Here's how the part is built. I have some questions about the finished solid (model axes, mm). Round coordinates to 2 decimals unless told otherwise and drop trailing zeros. Write each loop counter-clockwise with the first axis right and the second up, starting at its lowest first coordinate (ties: lowest second). Pieces come first, ordered by that corner, then holes. Notation, with made-up numbers: (46.25, -12) -> (92.25, -12) arc R19 cw to (92.25, 3) -> close; hole circle Ø5 at (60, 67.5). An arc over 180 degrees is marked (long way). Answer in a Markdown table with one row per item.
Autodesk Inventor part; units mm, degrees
ref_plane "YZ Plane" through (0, 0, 0) normal (1, 0, 0) x (0, 1, 0)
ref_plane "XZ Plane" through (0, 0, 0) normal (0, 1, 0) x (-1, 0, 0)
ref_plane "XY Plane" through (0, 0, 0) normal (0, 0, 1) x (1, 0, 0)
sketch "Sketch1" plane through (0, 0, 0) normal (0, 0, 1) x (1, 0, 0)
  line L0 (0, 0) -> (425, 0)
  line L1 (425, 0) -> (425, 300)
  line L2 (425, 300) -> (0, 300)
  line L3 (0, 300) -> (0, 0)
  line L4 (12.5, 287.5) -> (12.5, 12.5) construction
  line L5 (412.5, 287.5) -> (412.5, 12.5) construction
  point P0 (132.5, 270)
  point P1 (172.5, 270)
  point P2 (212.5, 270)
  point P3 (252.5, 270)
  point P4 (292.5, 270)
  point P5 (212.5, 300)
  dimension "d0" = 425
  dimension "d1" = 300
  dimension "d2" = 400
  dimension "d3" = 12.5
  dimension "d4" = 12.5
  dimension "d5" = 12.5
  dimension "d6" = 12.5
  dimension "d7" = 12.5
  dimension "d19" = 40
  dimension "d24" = 212.5
  dimension "d32" = 30
extrude "Extrusion1" add sketch "Sketch1" along normal blind 3
hole "Hole1" at (12.5, 287.5, 0) at (412.5, 287.5, 0) at (12.5, 12.5, 0) at (412.5, 12.5, 0) direction (0, 0, 1) diameter 6.4 end through all
hole "Hole2" at (132.5, 270, 0) at (172.5, 270, 0) at (212.5, 270, 0) at (252.5, 270, 0) at (292.5, 270, 0) direction (0, 0, 1) diameter 10 end through all
properties part number "back_wall"
1) For pin 1 (8 mm diameter, centred on x = 212.5, y = 270, fed in from +Z), with a flat end and sliding along its axis, tell me the tip position at first contact or that it passes through.
Response:
| item | result |
|---|---|
| pin 1 | passes through |
2) I need wall thicknesses on line 1 (X direction, y = 270, z = 2.1); line 2 (X direction, y = 12.5, z = 1.85); line 3 (Y direction, x = 412.5, z = 1.7). Which ranges of each line are inside material? Lowest first, please. Write a range as [from, to].
Response:
| item | result |
|---|---|
| line 1 | x = [0, 127.5], [137.5, 167.5], [177.5, 207.5], [217.5, 247.5], [257.5, 287.5], [297.5, 425] |
| line 2 | x = [0, 9.3], [15.7, 409.3], [415.7, 425] |
| line 3 | y = [0, 9.3], [15.7, 284.3], [290.7, 300] |
3) We'd pull the mould along X, two halves only. Please class faces 1 (the face through (210, 152, 0)), 2 (the face through (211, 274.77, 1.52)): +X half, -X half, draft (parallel to the pull), parting line (faces both ways), or undercut.
Response:
| item | result |
|---|---|
| face 1 | draft |
| face 2 | undercut |
4) I want a section at A-A, the plane x = 292.5. List the corners of the cut face in (y, z) for me, and give its area (3 significant figures).
Response:
| item | result |
|---|---|
| outline | (0, 0) -> (265, 0) -> (265, 3) -> (0, 3) -> close; (275, 0) -> (300, 0) -> (300, 3) -> (275, 3) -> close |
| area | 870 mm^2 |
